Here's how the part is built. I have some questions about the finished solid (model axes, mm). Round coordinates to 2 decimals unless told otherwise and drop trailing zeros. Write each loop counter-clockwise with the first axis right and the second up, starting at its lowest first coordinate (ties: lowest second). Pieces come first, ordered by that corner, then holes. Notation, with made-up numbers: M 82.25,70.25 L 104.25,70.25 A4 ccw 104.25,77.25 Z; hole C -38,83.25 d11. An arc over 180 degrees is marked long. Use a Markdown table: item, result. Add a question column.
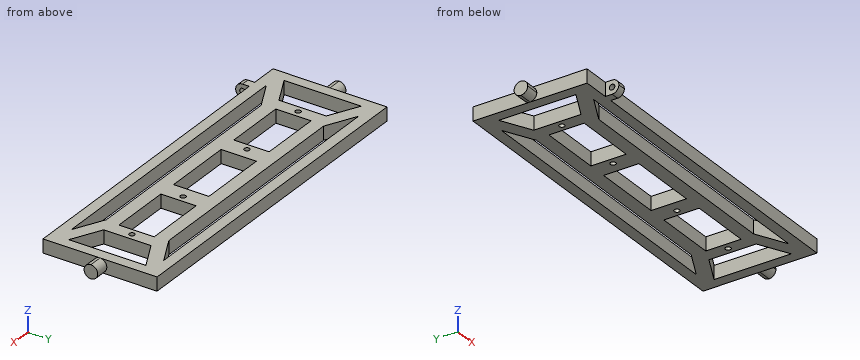
```python
from build123d import *

# Parameters (mm, degrees)
F0_W     = 126
F0_H     = 42
F0_R     = 1
F0_W_2   = 23
F0_H_2   = 13
F0_W_3   = 26
F1_DEPTH = 5
F3_DEPTH = 5
F4_W     = 3
F4_H     = 5
F5_DEPTH = 5
F6_R     = 1
F7_DEPTH = 3


# Not quite as in the source:
# - a pattern or mirror of a feature is missing from the dataset's text; its kind, count and spacing are read off the source's solid


with BuildPart() as f1:
    # F0 (on Top) → F1 (new body)
    with BuildSketch(Plane.XY):
        Rectangle(F0_W, F0_H)
        Polygon((-7, -11.5), (7, -11.5), (42.4098300563, -11.5), (53.4098300563, -17), (-53.4098300563, -17), (-42.4098300563, -11.5), align=None, mode=Mode.SUBTRACT)
        Polygon((-59, 14.2049150281), (-48, 8.7049150281), (-48, -8.7049150281), (-59, -14.2049150281), align=None, mode=Mode.SUBTRACT)
        with Locations((-45.5, 0)):
            Circle(F0_R, mode=Mode.SUBTRACT)
        with Locations((-31.5, 0)):
            Rectangle(F0_W_2, F0_H_2, mode=Mode.SUBTRACT)
        with Locations((-17.5, 0)):
            Circle(F0_R, mode=Mode.SUBTRACT)
        Rectangle(F0_W_3, F0_H_2, mode=Mode.SUBTRACT)
        with Locations((17.5, 0)):
            Circle(F0_R, mode=Mode.SUBTRACT)
        with Locations((31.5, 0)):
            Rectangle(F0_W_2, F0_H_2, mode=Mode.SUBTRACT)
        with Locations((45.5, 0)):
            Circle(F0_R, mode=Mode.SUBTRACT)
        Polygon((48, -8.7049150281), (48, 8.7049150281), (59, 14.2049150281), (59, -14.2049150281), align=None, mode=Mode.SUBTRACT)
        Polygon((42.4098300563, 11.5), (7, 11.5), (-7, 11.5), (-42.4098300563, 11.5), (-53.4098300563, 17), (53.4098300563, 17), align=None, mode=Mode.SUBTRACT)
    extrude(amount=F1_DEPTH)

    # F2 (on face) → F3 (join)
    with BuildSketch(Plane(origin=(-63, 0, 0), x_dir=(0, -1, 0), z_dir=(-1, 0, 0))):
        with BuildLine():
            ThreePointArc((0, 0), (1.767766953, 0.732233047), (2.5, 2.5))
            ThreePointArc((2.5, 2.5), (1.7677669583, 4.2677669477), (1.5e-08, 5))
            ThreePointArc((1.5e-08, 5), (-2.5, 2.5000000075), (0, 0))
        make_face()
    f3 = extrude(amount=F3_DEPTH)

    # F3_copies: F3 across plane
    add(f3.mirror(Plane(origin=(0, 0, 0), x_dir=(0, 0, 1), z_dir=(1, 0, 0))))

    # F4 (on face) → F5 (join)
    with BuildSketch(Plane.XZ.offset(21)):
        with Locations((-51.5, 2.5)):
            Rectangle(F4_W, F4_H)
    extrude(amount=F5_DEPTH)

    # F6 (on face) → F7 (cut, through all)
    with BuildSketch(Plane(origin=(-53, 0, 0), x_dir=(0, -1, 0), z_dir=(-1, 0, 0))):
        with Locations((23.5, 2.5)):
            Circle(F6_R)
        with BuildLine():
            Line((26, 2.5), (26, 5))
            Line((26, 5), (23.5, 5))
            ThreePointArc((23.5, 5), (25.267766953, 4.267766953), (26, 2.5))
        make_face()
        with BuildLine():
            Line((26, 0), (26, 2.5))
            ThreePointArc((26, 2.5), (25.267766953, 0.732233047), (23.5, 0))
            Line((23.5, 0), (26, 0))
        make_face()
    extrude(amount=-F7_DEPTH, mode=Mode.SUBTRACT)


solid = f1.part
```
Item 1: Imagine slicing it at A-A on x = -39. List the corners of the cut face in (y, z) for me, plus the area to 3 significant figures.
Item 2: I need wall thicknesses on probe 1 along Y at (x, z) = (-6, 2.85); probe 2 along Y at (x, z) = (14, 2.2); probe 3 along X at (y, z) = (-3, 3.85). Which ranges of each line are inside material? Lowest first, please. Write a range as from..to.
Item 3: For pin 1 Ø1.5 at (y, z) = (-17, 0.5) entering from -X; pin 2 Ø2.5 at (y, z) = (-24.5, 3.5) entering from +X; pin 3 Ø2 at (y, z) = (13, 0.5) entering from +X; pin 4 Ø2 at (x, y) = (41.5, 5) entering from -Z, each with a flat end and sliding along its axis, tell me the tip position at first contact or that it passes through.
The answers:
| question | item | result |
|---|---|---|
| 1 | outline | M -21,0 L -17,0 L -17,5 L -21,5 Z; M -11.5,0 L -6.5,0 L -6.5,5 L -11.5,5 Z; M 6.5,0 L 11.5,0 L 11.5,5 L 6.5,5 Z; M 17,0 L 21,0 L 21,5 L 17,5 Z |
| 1 | area | 90.0 mm² |
| 2 | probe 1 | -21..-17, -11.5..-6.5, 6.5..11.5, 17..21 |
| 2 | probe 2 | -21..-17, -11.5..11.5, 17..21 |
| 2 | probe 3 | -63..-59, -48..-43, -20..-13, 13..20, 43..48, 59..63 |
| 3 | pin 1 | x = -63 |
| 3 | pin 2 | x = -50 |
| 3 | pin 3 | x = 63 |
| 3 | pin 4 | through |
